from build123d import *

# Parameters (mm, degrees)
EXTRUDE_1_DEPTH     = 22
SKETCH_2_W          = 5
SKETCH_2_H          = 1.8
SKETCH_2_W_2        = 7
SKETCH_2_H_2        = 2.3
CUT_EXTRUDE_1_DEPTH = 4
CUT_EXTRUDE_2_DEPTH = 64.319089808
SKETCH_3_3_R        = 14
EXTRUDE_2_DEPTH     = 0.3
SKETCH_4_W          = 4.8
SKETCH_4_H          = 4.8
EXTRUDE_3_DEPTH     = 0.8
SKETCH_5_R          = 0.85
CUT_EXTRUDE_3_DEPTH = 63.897702188
SKETCH_6_W          = 11
SKETCH_6_H          = 2
CUT_EXTRUDE_4_DEPTH = 1
SKETCH_7_W          = 4.8
SKETCH_7_H          = 4.8
EXTRUDE_4_DEPTH     = 0.8


with BuildPart() as part:
    # Sketch 1 → Extrude 1 (new body)
    with BuildSketch(Plane(origin=(0, 0, 0), x_dir=(0, 0, -1), z_dir=(1, 0, 0))):
        with BuildLine():
            Line((0, -25), (0, -2))
            ThreePointArc((0, -2), (0.585786438, -0.585786438), (2, 0))
            Line((2, 0), (23.64572618, 0))
            ThreePointArc((23.64572618, 0), (23.99456936, -0.030657867), (24.332717753, -0.121691565))
            Line((24.332717753, -0.121691565), (52.174626532, -10.304873595))
            Line((52.174626532, -10.304873595), (52.277675268, -10.023127329))
            Line((52.277675268, -10.023127329), (24.435766489, 0.160054701))
            ThreePointArc((24.435766489, 0.160054701), (24.046895837, 0.264743453), (23.64572618, 0.3))
            Line((23.64572618, 0.3), (2, 0.3))
            ThreePointArc((2, 0.3), (0.373654403, -0.373654403), (-0.3, -2))
            Line((-0.3, -2), (-0.3, -25))
            Line((-0.3, -25), (0, -25))
        make_face()
    extrude(amount=EXTRUDE_1_DEPTH)

    # Sketch 2 → Cut-Extrude 1 (cut)
    with BuildSketch(Plane.XY.offset(0.3)):
        with Locations((8.5, -0.9)):
            Rectangle(SKETCH_2_W, SKETCH_2_H)
        with Locations((13.5, -0.9)):
            Rectangle(SKETCH_2_W, SKETCH_2_H)
        with Locations((7.5, -3.15)):
            Rectangle(SKETCH_2_W_2, SKETCH_2_H_2)
        with Locations((14.5, -3.15)):
            Rectangle(SKETCH_2_W_2, SKETCH_2_H_2)
        Polygon((4, -1.8), (4, -2), (11, -2), (11, -1.8), (6, -1.8), align=None)
        Polygon((11, -1.8), (11, -2), (18, -2), (18, -1.8), (16, -1.8), align=None)
    extrude(amount=-CUT_EXTRUDE_1_DEPTH, mode=Mode.SUBTRACT)

    # Sketch 3 → Cut-Extrude 2 (cut, through all)
    with BuildSketch(Plane(origin=(0, 8.024038665, -2.934793264), x_dir=(1, 0, 0), z_dir=(0, 0.9391542177229502, -0.3434957864853564))):
        with BuildLine():
            ThreePointArc((13.196152423, 52.539701225), (19.591939741, 47.38998358), (22, 39.539701225))
            Line((22, 39.539701225), (22, 52.539701225))
            Line((22, 52.539701225), (13.196152423, 52.539701225))
        make_face()
        with BuildLine():
            ThreePointArc((0, 51.028826518), (1.358818231, 51.864258204), (2.803847577, 52.539701225))
            Line((2.803847577, 52.539701225), (0, 52.539701225))
            Line((0, 52.539701225), (0, 51.028826518))
        make_face()
    extrude(amount=-CUT_EXTRUDE_2_DEPTH, mode=Mode.SUBTRACT)

    # Sketch 3_3 → Extrude 2 (add)
    with BuildSketch(Plane(origin=(0, 8.024038665, -2.934793264), x_dir=(1, 0, 0), z_dir=(0, 0.9391542177229502, -0.3434957864853564))):
        with Locations((8, 39.539701225)):
            Circle(SKETCH_3_3_R)
    extrude(amount=-EXTRUDE_2_DEPTH)

    # Sketch 4 → Extrude 3 (add)
    with BuildSketch(Plane.XY.offset(0.3)):
        with Locations((11, -9.75)):
            Rectangle(SKETCH_4_W, SKETCH_4_H)
        with Locations((11, -21.05)):
            Rectangle(SKETCH_4_W, SKETCH_4_H)
        with Locations((5.35, -15.4)):
            Rectangle(SKETCH_4_W, SKETCH_4_H)
        with Locations((16.65, -15.4)):
            Rectangle(SKETCH_4_W, SKETCH_4_H)
    extrude(amount=EXTRUDE_3_DEPTH)

    # Sketch 5 → Cut-Extrude 3 (cut, through all)
    with BuildSketch(Plane(origin=(0, 0.3, 0), x_dir=(1, 0, 0), z_dir=(0, 1, 0))):
        with Locations(Location((8, 7.64572618, 0), (0, 0, 270))):
            Circle(SKETCH_5_R)
        with Locations(Location((14, 7.64572618, 0), (0, 0, 270))):
            Circle(SKETCH_5_R)
    extrude(amount=-CUT_EXTRUDE_3_DEPTH, mode=Mode.SUBTRACT)

    # Sketch 6 → Cut-Extrude 4 (cut)
    with BuildSketch(Plane(origin=(0, 8.024038665, -2.934793264), x_dir=(1, 0, 0), z_dir=(0, 0.9391542177229502, -0.3434957864853564))):
        with Locations((11, 23.2)):
            Rectangle(SKETCH_6_W, SKETCH_6_H)
    extrude(amount=-CUT_EXTRUDE_4_DEPTH, mode=Mode.SUBTRACT)

    # Sketch 7 → Extrude 4 (add)
    with BuildSketch(Plane(origin=(0, 8.024038665, -2.934793264), x_dir=(1, 0, 0), z_dir=(0, 0.9391542177229502, -0.3434957864853564))):
        with Locations((9.738477049, 36.851443585)):
            Rectangle(SKETCH_7_W, SKETCH_7_H)
        with Locations((14.118767038, 47.774445204)):
            Rectangle(SKETCH_7_W, SKETCH_7_H)
        with Locations((5.219570287, 48.855656024)):
            Rectangle(SKETCH_7_W, SKETCH_7_H)
        with Locations((-1.489481468, 43.037611303)):
            Rectangle(SKETCH_7_W, SKETCH_7_H)
        with Locations((-1.651961899, 34.079108149)):
            Rectangle(SKETCH_7_W, SKETCH_7_H)
    extrude(amount=EXTRUDE_4_DEPTH)


solid = part.part
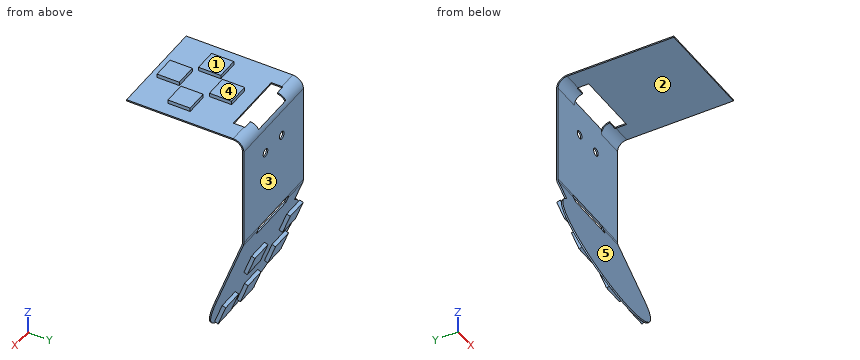
The model under review builds one solid part; all positions refer to its coordinate system, in mm. Face numbers are marked on the shaded views. A direction names the side the tool comes from. Coordinates: 2 decimals unless noted, no trailing zeros. Write each loop counter-clockwise with the first axis right and the second up, starting at its lowest first coordinate (ties: lowest second). Pieces come first, ordered by that corner, then holes. Notation, with made-up numbers: (-13, -2) - (20, -2) arc R21 ccw to (20, 35) - close; hole circle Ø4 at (-34, 25). An arc over 180 degrees is marked (long way). Answer as a JSON object with one key per item and string values. Group by question number.
1. Add section A-A (x = 9.5). Give the boundary of the cut face in (y, z).
2. Mouldability with a two-part tool opening along Z and no side actions: class the marked faces 1, 2 and 3 as pulls with the +Z half, pulls with the -Z half, needs draft (parallel to the pull), parting line crosses it, or undercut.
3. To check wall thickness, follow probe 1 along Z at (x, y) = (2.5, -17.75); probe 2 along Z at (x, y) = (12.5, -22). State the ranges of each line that lie inside material, in increasing order.
4. Clearance check with flat-ended pins moving along their axes: pin 1 Ø8 at (x, y) = (3.5, -13.5) entering from -Z; pin 2 Ø2.5 at (y, z) = (-7.5, -47.5) entering from +X; pin 3 Ø2 at (x, z) = (12.5, -38.5) entering from -Y; pin 4 Ø2.5 at (y, z) = (-5, -36.5) entering from +X. State where each tip first meets the part, or that it passes through.
5. Machinability: for the marked faces 4 and 5, which of the approach directions +Z, -Z, +X, -X, +Y, -Y give a long, thin tool a straight path to every point of the face, cutting with its end or side? Answer none if there is none.
6. Add section C-C (z = -14). Give the boundary of the cut face in (x, y), plus the area to 3 significant figures.
7. Add section B-B (x = 20.25). Give the boundary of the cut face in (y, z).
Findings:
{
 "1": {"outline": "(-25, 0) - (-4.3, 0) - (-4.3, 0.3) - (-7.35, 0.3) - (-7.35, 1.1) - (-12.15, 1.1) - (-12.15, 0.3) - (-18.65, 0.3) - (-18.65, 1.1) - (-23.45, 1.1) - (-23.45, 0.3) - (-25, 0.3) - close; (-10.62, -53.04) - (-10.34, -53.14) - (-5.46, -39.8) - (-4.71, -40.07) - (-3.06, -35.56) - (-3.81, -35.29) - (-0.29, -25.66) - (-0.57, -25.56) - close; (0, -23.64) - (0.3, -23.75) arc R2.3 ccw to (0.3, -23.65) - (0.3, -2) arc R2.3 ccw to (0, -0.86) - close"},
 "2": {"face 1": "pulls with the +Z half", "face 2": "undercut", "face 3": "needs draft"},
 "3": {"probe 1": "0 to 0.3", "probe 2": "0 to 1.1"},
 "4": {"pin 1": "z = -53.07", "pin 2": "x = 20.33", "pin 3": "y = -5.67", "pin 4": "x = 22"},
 "5": {"face 4": "+Z, +X, -X, +Y, -Y", "face 5": "+X, -X, -Y"},
 "6": {"outline": "(0, 0) - (22, 0) - (22, 0.3) - (0, 0.3) - close", "area": "6.60 mm²"},
 "7": {"outline": "(-25, 0) - (-2, 0) arc R2 cw to (0, -2) - (0, -23.65) arc R2 cw to (-0.12, -24.33) - (-8.17, -46.33) - (-7.89, -46.43) - (0.16, -24.44) arc R2.3 ccw to (0.3, -23.65) - (0.3, -2) arc R2.3 ccw to (-2, 0.3) - (-25, 0.3) - close"}
}
